For this review, take the finished solid that the model builds, in its own axes (mm). A direction names the side the tool comes from. Give positions to 0.01 mm unless a question says otherwise; leave off trailing zeros. Write each loop counter-clockwise with the first axis right and the second up, starting at its lowest first coordinate (ties: lowest second). Pieces come first, ordered by that corner, then holes. Notation, with made-up numbers: M 40.25,13 L 69.25,13 A23 cw 69.25,38 Z; hole C 33,16.5 d10. An arc over 180 degrees is marked long. Answer as a JSON object with one key per item and string values. Group by question number.
Autodesk Inventor part; units mm, degrees
ref_plane "YZ Plane" through (0, 0, 0) normal (1, 0, 0) x (0, 1, 0)
ref_plane "XZ Plane" through (0, 0, 0) normal (0, 1, 0) x (-1, 0, 0)
ref_plane "XY Plane" through (0, 0, 0) normal (0, 0, 1) x (1, 0, 0)
sketch "Sketch1" plane through (0, 0, 0) normal (0, 1, 0) x (-1, 0, 0)
  line L0 (-15, 12.25) -> (15, 12.25)
  line L1 (15, 12.25) -> (15, -12.25)
  line L2 (15, -12.25) -> (-15, -12.25)
  line L3 (-15, -12.25) -> (-15, 12.25)
  line L4 (-15, 12.25) -> (15, -12.25) construction
  line L5 (15, 12.25) -> (-15, -12.25) construction
  line L6 (-12, 12.25) -> (12, 12.25)
  line L7 (12, 12.25) -> (12, -12.25)
  line L8 (12, -12.25) -> (-12, -12.25)
  line L9 (-12, -12.25) -> (-12, 12.25)
  line L10 (-12, 12.25) -> (12, -12.25) construction
  line L11 (12, 12.25) -> (-12, -12.25) construction
  circle A0 centre (12, -12.25) radius 1.25
  circle A1 centre (-12, -12.25) radius 1.25
  circle A2 centre (-12, 12.25) radius 1.25
  circle A3 centre (12, 12.25) radius 1.25
  point P0 (0, 0)
  point P1 (13.25, 12.25)
  point P2 (10.75, 12.25)
  point P3 (-10.75, 12.25)
  point P4 (-13.25, 12.25)
  point P5 (-13.25, -12.25)
  point P6 (-10.75, -12.25)
  point P7 (10.75, -12.25)
  point P8 (13.25, -12.25)
  dimension "d0" = 30
  dimension "d1" = 24.5
  dimension "d2" = 24
  dimension "d3" = 2.5
extrude "Extrusion1" add sketch "Sketch1" along normal blind 1 contours L0 A3 L7 A0 L2 A1 L9 A2 | A2 L9 A1 L2 L3 L0 | L0 L1 L2 A0 L7 A3
sketch "Sketch2" plane through (0, 1, 0) normal (0, 1, 0) x (1, 0, 0)
  line L0 (-6.3, 6.3) -> (6.3, 6.3)
  line L1 (6.3, 6.3) -> (6.3, -6.3)
  line L2 (6.3, -6.3) -> (-6.3, -6.3)
  line L3 (-6.3, -6.3) -> (-6.3, 6.3)
  line L4 (-6.3, 6.3) -> (6.3, -6.3) construction
  line L5 (6.3, 6.3) -> (-6.3, -6.3) construction
  point P0 (0, 0)
  dimension "d6" = 12.6
  dimension "d7" = 12.6
extrude "Extrusion2" add sketch "Sketch2" along normal blind 3
sketch "Sketch3" plane through (0, 4, 0) normal (0, 1, 0) x (1, 0, 0)
  circle A0 centre (0, 0) radius 6.75
  dimension "d10" = 13.5
extrude "Extrusion3" add sketch "Sketch3" along normal blind 3.5 and the other way blind 3
properties part number "Camera"
Item 1: To check wall thickness, follow probe 1 along Y at (x, z) = (-4.25, 8); probe 2 along Z at (x, y) = (0.25, 3); probe 3 along X at (y, z) = (3.75, -3). State the ranges of each line that lie inside material, in increasing order.
Item 2: Consider section B-B (y = 3.25). Give the boundary of the cut face in (x, z).
Item 3: Draft analysis for pull direction X (two halves, no side actions). For faces 5 (the cylindrical face through (12, 0.5, 11)), 6 (the flat face through (-14.1, 0.5, -12.25)), 7 (the cylindrical face through (-4.975, 4.927, 4.562)), state which applies: released by +X, released by -X, zero draft, split by the parting line, or undercut.
Item 4: Insertion check: P1, Ø1.5, axis at x = 4, y = 2, coming from the +Z side; P2, Ø0.9, axis at x = 4, y = 2, coming from the -Z side; P3, Ø1.5, axis at y = 2.5, z = 1, coming from the +X side. Each pin has a flat end and moves straight along its axis. Give the tip position at first contact, or say it passes through.
Item 5: Machinability: for faces 1 (the flat face through (-5, 4, -5)), 2 (the flat face through (4, 2, 6.3)), 3 (the flat face through (4, 2, -6.3)), 4 (the flat face through (-6.3, 2, 4)), which of the approach directions +Z, -Z, +X, -X, +Y, -Y give a long, thin tool a straight path to every point of the face, cutting with its end or side? Answer none if there is none.
Item 6: Consider section A-A (x = 0). Give the boundary of the cut face in (y, z).
Item 7: Consider section C-C (z = 0). Give the boundary of the cut face in (x, y).
Item 8: Consider section D-D (y = 6). Give the boundary of the cut face in (x, z), plus the area to 3 significant figures.
Result set:
{
 "1": {"probe 1": "y = 0 to 1", "probe 2": "z = -6.75 to 6.75", "probe 3": "x = -6.3 to 6.3"},
 "2": {"outline": "M -6.3,-6.3 L -2.42,-6.3 A6.75 ccw 2.42,-6.3 L 6.3,-6.3 L 6.3,-2.42 A6.75 ccw 6.3,2.42 L 6.3,6.3 L 2.42,6.3 A6.75 ccw -2.42,6.3 L -6.3,6.3 L -6.3,2.42 A6.75 ccw -6.3,-2.42 Z"},
 "3": {"face 5": "undercut", "face 6": "zero draft", "face 7": "split by the parting line"},
 "4": {"P1": "stops at z = 6.3", "P2": "stops at z = -6.3", "P3": "stops at x = 6.75"},
 "5": {"face 1": "-Z, -X, +Y", "face 2": "+Z, +X, +Y", "face 3": "-Z, +X, +Y", "face 4": "+Z, -X, +Y"},
 "6": {"outline": "M 0,-12.25 L 1,-12.25 L 1,-6.75 L 7.5,-6.75 L 7.5,6.75 L 1,6.75 L 1,12.25 L 0,12.25 Z"},
 "7": {"outline": "M -15,0 L 15,0 L 15,1 L 6.75,1 L 6.75,7.5 L -6.75,7.5 L -6.75,1 L -15,1 Z"},
 "8": {"outline": "C 0,0 d13.5", "area": "143 mm^2"}
}
